Check sheet for the modelled part. Datum: model origin and axes. Units: mm. Coordinates: 2 decimals unless noted, no trailing zeros. Order: outer loops, then holes, each group sorted by start corner. A loop starts at its lowest first (then second) coordinate and runs counter-clockwise, first axis right, second up. Notation, with made-up numbers: (-23, -5.5) -> (17, -5.5) arc R25 ccw to (17, 12.5) -> close; hole circle Ø11 at (-27.75, 33.25). An arc over 180 degrees is marked (long way). Put each result on its own line as item: value. Start each with the question number.
```python
from build123d import *

# Parameters (mm, degrees)
VYSUNOUT1_DEPTH = 1
ZKOSIT1_SIZE    = 0.25


with BuildPart() as part:
    # Skica1 → Vysunout1 (new, symmetric)
    with BuildSketch(Plane(origin=(0, 0, 0), x_dir=(1, 0, 0), z_dir=(0, 1, 0))):
        with BuildLine():
            Line((-1, 3), (-1, -3))
            ThreePointArc((-1, -3), (0, -4), (1, -3))
            Line((1, -3), (1, 3))
            ThreePointArc((1, 3), (0, 4), (-1, 3))
        make_face()
    extrude(amount=VYSUNOUT1_DEPTH, both=True)

    # Zkosit1
    zkosit1_edges = [part.edges().sort_by_distance(p)[0] for p in [
        (0, 1, 4),
        (1, 1, 0),
        (0, 1, -4),
        (1, -1, 0),
        (0, -1, 4),
        (-1, -1, 0),
        (0, -1, -4),
        (-1, 1, 0),
    ]]
    chamfer(zkosit1_edges, length=ZKOSIT1_SIZE)


solid = part.part
```
1) Sectioned sample at A-A (z = 2.5). Record the boundary of the cut face in (x, y).
2) Sectioned sample at B-B (y = 0.85). Record the boundary of the cut face in (x, z), plus the area to 3 significant figures.
3) Scan lines: line 1 along Z through (x, y) = (-0.05, 0.2); line 2 along Z through (x, y) = (0.65, -0.5); line 3 along Y through (x, z) = (-0.6, 3.5). Record each from-to range of solid material in increasing order. Write a range as [from, to].
Entries:
1. outline: (-1, -0.75) -> (-0.75, -1) -> (0.75, -1) -> (1, -0.75) -> (1, 0.75) -> (0.75, 1) -> (-0.75, 1) -> (-1, 0.75) -> close
2. outline: (-0.9, -3) arc R0.9 ccw to (0.9, -3) -> (0.9, 3) arc R0.9 ccw to (-0.9, 3) -> close
2. area: 13.3 mm2
3. line 1: z = [-4, 4]
3. line 2: z = [-3.76, 3.76]
3. line 3: y = [-0.97, 0.97]
